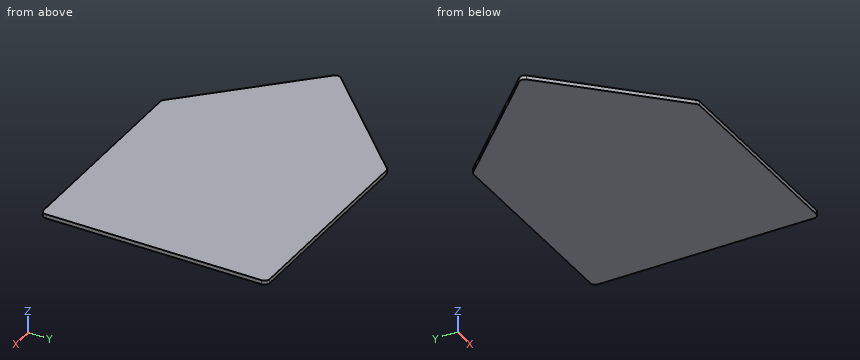
Autodesk Inventor part; units mm, degrees
ref_plane "YZ Plane" through (0, 0, 0) normal (1, 0, 0) x (0, 1, 0)
ref_plane "XZ Plane" through (0, 0, 0) normal (0, 1, 0) x (-1, 0, 0)
ref_plane "XY Plane" through (0, 0, 0) normal (0, 0, 1) x (1, 0, 0)
sketch "Sketch1" plane through (0, 0, 0) normal (0, 0, 1) x (1, 0, 0)
  line L0 (-20.5, 22) -> (20.5, 22)
  line L1 (20.5, 22) -> (20.5, -22)
  line L2 (20.5, -22) -> (-20.5, -22)
  line L3 (-20.5, -22) -> (-20.5, 22) construction
  line L4 (-20.5, 22) -> (20.5, -22) construction
  line L5 (-20.5, -22) -> (-42.5, 0)
  line L6 (-42.5, 0) -> (-20.5, 22)
  point P0 (0, 0)
  point P1 (0, 0)
  point P2 (20.5, 0)
  dimension "d0" = 41
  dimension "d1" = 44
  dimension "d4" = 63
extrude "Plate1" add sketch "Sketch1" along normal blind 0.8
fillet "Corner Round2" radius 1 5 edges at (-20.5, -22, 0.4) (-42.5, 0, 0.4) (-20.5, 22, 0.4) (20.5, -22, 0.4) (20.5, 22, 0.4)
equation "\"d2\" = Thickness"
equation "\"BendReliefWidth\" = Thickness"
equation "\"BendReliefDepth\" = 0.5 * Thickness"
equation "\"CornerReliefSize\" = 4 * Thickness"
equation "\"MinimumRemnant\" = 2 * Thickness"
equation "\"TransitionRadius\" = BendRadius"
equation "\"JacobiRadiusSize\" = BendRadius"
equation "\"GapSize\" = Thickness"
properties part number "MNT-CDF-604 CAP" material "Stainless Steel"
Here's how the part is built. I have some questions about the finished solid (model axes, mm). Coordinates: 2 decimals unless noted, no trailing zeros. Order: outer loops, then holes, each group sorted by start corner. A loop starts at its lowest first (then second) coordinate and runs counter-clockwise, first axis right, second up. Notation, with made-up numbers: (-32.75, -31.75) - (0.25, -31.75) arc R30 ccw to (0.25, 1.25) - close; hole circle Ø11 at (38, -22). An arc over 180 degrees is marked (long way). Use CSV: the item, a comma, the result in double quotes. Start each with the question number.
1. Suppose I cut it at A-A on z = 0.55. List the corners of the cut face in (x, y) for me.
2. Suppose I cut it at B-B on y = -17. List the corners of the cut face in (x, z) for me.
3. Please list where these lines run through material, in increasing order: line 1 (Y direction, x = -24.5, z = 0.6); line 2 (X direction, y = -12, z = 0.7); line 3 (X direction, y = 6.5, z = 0.7). Write a range as from..to.
4. Suppose I cut it at C-C on x = -36. List the corners of the cut face in (y, z) for me, then the cut area to 3 significant figures.
5. I'm going to push a flat-ended pin straight in: pin 1 (12 mm diameter, centred on x = -28.5, y = -15, fed in from -Z). Where does the tip first touch, or does it pass through?
Output:
1,outline,"(-41.79, -0.71) - (-20.79, -21.71) arc R1 ccw to (-20.09, -22) - (19.5, -22) arc R1 ccw to (20.5, -21) - (20.5, 21) arc R1 ccw to (19.5, 22) - (-20.09, 22) arc R1 ccw to (-20.79, 21.71) - (-41.79, 0.71) arc R1 ccw to start"
2,outline,"(-25.5, 0) - (20.5, 0) - (20.5, 0.8) - (-25.5, 0.8) - close"
3,line 1,"y = -18..18"
3,line 2,"x = -30.5..20.5"
3,line 3,"x = -36..20.5"
4,outline,"(-6.5, 0) - (6.5, 0) - (6.5, 0.8) - (-6.5, 0.8) - close"
4,area,"10.4 mm2"
5,pin 1,"stops at z = 0"
